Input: part model. Units: mm. Frame: model coordinates. A direction names the side the tool comes from. Give positions to 0.01 mm unless a question says otherwise; leave off trailing zeros. Loops run counter-clockwise (first coordinate to the right, second up) from the corner with the lowest first, then second, coordinate; pieces in that order, holes last. Notation, with made-up numbers: (47.25, 11.5) - (92.25, 11.5) arc R18 cw to (92.25, 26.5) - close; hole circle Ø2 at (69, 70). An arc over 180 degrees is marked (long way). One line per item, written item: value.
from build123d import *

# Parameters (mm, degrees)
SKETCH1_R           = 1.6
BOSS_EXTRUDE1_DEPTH = 5
CUT_EXTRUDE1_START  = -3
SKETCH2_R           = 1.6
CUT_EXTRUDE1_DEPTH  = 3


with BuildPart() as part:
    # Sketch1 → Boss-Extrude1 (new body)
    with BuildSketch(Plane.XY):
        with BuildLine():
            ThreePointArc((31.466251763, 27.930717857), (33.905409352, 33.905409352), (27.930717857, 31.466251763))
            Line((27.930717857, 31.466251763), (11.985099135, 15.520633041))
            ThreePointArc((11.985099135, 15.520633041), (9.545941546, 9.545941546), (15.520633041, 11.985099135))
            Line((15.520633041, 11.985099135), (31.466251763, 27.930717857))
        make_face()
        with Locations((31.430535617, 31.430535617)):
            Circle(SKETCH1_R, mode=Mode.SUBTRACT)
        with Locations((12.02081528, 12.02081528)):
            Circle(SKETCH1_R, mode=Mode.SUBTRACT)
    extrude(amount=BOSS_EXTRUDE1_DEPTH)

    # Sketch2 → Cut-Extrude1 (cut)
    # profile 1 of 2: a face of its own
    with BuildSketch(Plane.XY.offset(5).offset(CUT_EXTRUDE1_START)):
        with BuildLine():
            ThreePointArc((11.985099135, 15.520633041), (9.545941546, 9.545941546), (15.520633041, 11.985099135))
            Line((15.520633041, 11.985099135), (15.62569954, 12.090165634))
            Line((15.62569954, 12.090165634), (14.878553313, 14.878553313))
            Line((14.878553313, 14.878553313), (12.090165634, 15.62569954))
            Line((12.090165634, 15.62569954), (11.985099135, 15.520633041))
        make_face()
        with Locations((12.02081528, 12.02081528)):
            Circle(SKETCH2_R, mode=Mode.SUBTRACT)
    # profile 2 of 2: a face of its own
    with BuildSketch(Plane.XY.offset(5).offset(CUT_EXTRUDE1_START)):
        with BuildLine():
            Line((28.572797584, 28.572797584), (31.361185263, 27.825651357))
            Line((31.361185263, 27.825651357), (31.466251763, 27.930717857))
            ThreePointArc((31.466251763, 27.930717857), (33.905409352, 33.905409352), (27.930717857, 31.466251763))
            Line((27.930717857, 31.466251763), (27.825651357, 31.361185263))
            Line((27.825651357, 31.361185263), (28.572797584, 28.572797584))
        make_face()
        with Locations((31.430535617, 31.430535617)):
            Circle(SKETCH2_R, mode=Mode.SUBTRACT)
    extrude(amount=CUT_EXTRUDE1_DEPTH, mode=Mode.SUBTRACT)


solid = part.part
Item 1: Draft query along X for faces 4 (the face through (32.1, 29.8, 2)), 5 (the face through (29.947, 28.204, 3.479)), 6 (the face through (12.88, 13.37, 0.99)). Return one class per face: pulls with the +X half, pulls with the -X half, needs draft (parallel to the pull), parting line crosses it, or undercut.
Verdict:
face 4: needs draft
face 5: pulls with the +X half
face 6: undercut
Item 2: Section C-C, the plane y = 30.25. Output: boundary loops of the cut face in (x, z).
Verdict:
outline: (26.71, 0) - (30.35, 0) - (30.35, 2) - (28.12, 2) - (28.12, 5) - (26.71, 5) - close; (32.51, 0) - (34.73, 0) - (34.73, 2) - (32.51, 2) - close
Item 3: Pin query (flat end, axial travel): P1, Ø1.9, axis at x = 31.43, y = 31.43, coming from the -Z side; P2, Ø6, axis at x = 30.5, y = 23, coming from the +Z side; P3, Ø2, axis at y = 15.5, z = 2, coming from the -X side; P4, Ø1, axis at y = 17.5, z = 0.5, coming from the +X side. Return the tip coordinate at first contact, or that it passes through.
Verdict:
P1: passes through
P2: stops at z = 5
P3: stops at x = 9.55
P4: stops at x = 21.54
Item 4: Section B-B, the plane z = 3.35. Output: boundary loops of the cut face in (x, y), and give its area (3 significant figures).
Verdict:
outline: (12.09, 15.63) - (14.88, 14.88) - (15.63, 12.09) - (31.36, 27.83) - (28.57, 28.57) - (27.83, 31.36) - close
area: 104 mm^2
Item 5: Section A-A, the plane x = 32. Output: boundary loops of the cut face in (y, z).
Verdict:
outline: (27.98, 0) - (29.94, 0) - (29.94, 2) - (27.98, 2) - close; (32.93, 0) - (34.88, 0) - (34.88, 2) - (32.93, 2) - close
Item 6: Material intervals for L1, parallel to Z at x = 15, y = 11.5; L2, parallel to Y at x = 31.5, z = 0.7; L3, parallel to X at y = 31.25, z = 0.8, sorted ascending.
Verdict:
L1: z = 0 to 2
L2: y = 27.93 to 29.83, 33.03 to 34.93
L3: x = 27.71 to 29.84, 33.02 to 34.93
Item 7: Access query for faces 1 (the face through (14, 11, 2)), 2 (the face through (32.9, 30.8, 1)), 3 (the face through (28.194, 29.987, 3.479)). Directions: +Z, -Z, +X, -X, +Y, -Y. A direction counts if a zero-diameter tool reaches every point of the face in a straight line with its end or side. Return the directions, or none.
Verdict:
face 1: +Z, -X, -Y
face 2: +Z, -Z
face 3: +Z, +X, +Y
Item 8: Section D-D, the plane x = 11.25. Output: boundary loops of the cut face in (y, z), and give its area (3 significant figures).
Verdict:
outline: (8.61, 0) - (10.62, 0) - (10.62, 2) - (8.61, 2) - close; (13.42, 0) - (15.43, 0) - (15.43, 2) - (13.42, 2) - close
area: 8.05 mm^2
